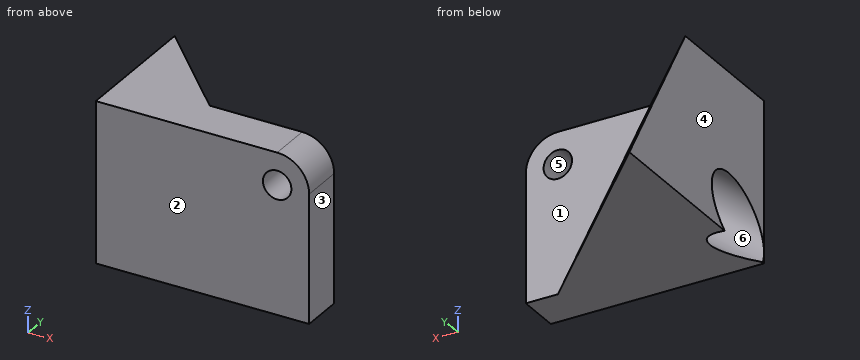
```python
from build123d import *

# Parameters (mm, degrees)
SKETCH_1_R          = 4
EXTRUDE_1_DEPTH     = 12
EXTRUDE_2_DEPTH     = 55
CUT_EXTRUDE_1_DEPTH = 50
SKETCH_9_R          = 9
CUT_EXTRUDE_2_DEPTH = 74.567594408


with BuildPart() as part:
    # 草图1 → 凸台-拉伸1 (new body)
    with BuildSketch(Plane(origin=(0, 0, 0), x_dir=(1, 0, 0), z_dir=(0, 1, 0))):
        with BuildLine():
            Line((-30, 22.5), (30, 22.5))
            Line((30, 22.5), (30, -13.5))
            ThreePointArc((30, -13.5), (27.363961031, -19.863961031), (21, -22.5))
            Line((21, -22.5), (-30, -22.5))
            Line((-30, -22.5), (-30, 22.5))
        make_face()
        with Locations(Location((21, -13.5, 0), (0, 0, 270))):
            Circle(SKETCH_1_R, mode=Mode.SUBTRACT)
    extrude(amount=EXTRUDE_1_DEPTH)

    # 草图5 → 凸台-拉伸2 (add)
    with BuildSketch(Plane(origin=(0, 12, 0), x_dir=(1, 0, 0), z_dir=(0, 1, 0))):
        Polygon((-5, -22.5), (20.980762114, 22.5), (-30, 22.5), (-30, -22.5), align=None)
    extrude(amount=EXTRUDE_2_DEPTH)

    # 草图6 → 切除-拉伸1 (cut)
    with BuildSketch(Plane(origin=(8.633922254, 8.365483215, 4.984797338), x_dir=(0.4999999999999977, 0, -0.86602540378444), z_dir=(-0.6634139481689368, -0.642787609686543, -0.3830222215594858))):
        Polygon((-21.985571585, -4.744524705), (29.975952642, -4.744524705), (46.861281787, -7.759213518), (18.600754365, -97.120116912), (-55.184549729, -73.785397471), align=None)
    extrude(amount=-CUT_EXTRUDE_1_DEPTH, mode=Mode.SUBTRACT)

    # 草图9 → 切除-拉伸2 (cut, through all)
    with BuildSketch(Plane(origin=(8.633922254, 8.365483215, 4.984797338), x_dir=(0.27508013503084955, 0.2665275624016649, -0.9237391286459811), z_dir=(0.663413948168937, 0.6427876096865428, 0.38302222155948573))):
        with Locations(Location((9.830913468, 29.914425108, 0), (0, 0, 90))):
            Circle(SKETCH_9_R)
    extrude(amount=-CUT_EXTRUDE_2_DEPTH, mode=Mode.SUBTRACT)


solid = part.part
```
Input: part model. Units: mm. Frame: model coordinates. Face numbers are marked on the shaded views. A direction names the side the tool comes from. Round coordinates to 2 decimals unless told otherwise and drop trailing zeros. Loops run counter-clockwise (first coordinate to the right, second up) from the corner with the lowest first, then second, coordinate; pieces in that order, holes last. Notation, with made-up numbers: M 50,81.5 L 101,81.5 A20 cw 101,108.5 Z; hole C -25,-1 d8. An arc over 180 degrees is marked long. Answer in a Markdown table with one row per item. Add a question column.
1. Ray query, probe 1 along X at (y, z) = (2.5, 13.5); probe 2 along Y at (x, z) = (25.5, 11); probe 3 along Z at (x, y) = (23.5, 3). Return the intervals inside material, ascending.
2. Section A-A (z = 5.5). Output: boundary loops of the cut face in (x, y), and give its area (3 significant figures).
3. Section B-B (y = 42). Output: boundary loops of the cut face in (x, z).
4. Contact query for flat-ended pins moving along their axis: pin 1 (5 mm diameter, centred on y = 7, z = -17.5, fed in from -X); pin 2 (4 mm diameter, centred on y = 27, z = -5.5, fed in from +X); pin 3 (8 mm diameter, centred on x = 8.5, z = -4, fed in from +Y). Output: stop coordinate, or through.
5. Mould query, pull axis X, two halves, no side actions, for the marked faces 3, 4, 5 and 6. Classes: released by +X, released by -X, zero draft, split by the parting line, or undercut.
6. Set-up query: the marked faces 1 and 2. Return all of +Z, -Z, +X, -X, +Y, -Y with unobstructed straight access to the full face (end or side cutting, diameter ignored); none if empty.
Values follow:
| question | item | result |
|---|---|---|
| 1 | probe 1 | -30 to 17, 25 to 30 |
| 1 | probe 2 | 0 to 12 |
| 1 | probe 3 | -22.5 to 10.38, 16.62 to 22.15 |
| 2 | outline | M -30,0 L 30,0 L 30,12 L 4.81,12 L -30,47.93 Z |
| 2 | area | 1,350 mm^2 |
| 3 | outline | M -30,-22.5 L -8.09,-22.5 L -30,15.46 Z |
| 4 | pin 1 | x = -25.45 |
| 4 | pin 2 | x = -1.11 |
| 4 | pin 3 | y = 18.62 |
| 5 | face 3 | released by +X |
| 5 | face 4 | released by -X |
| 5 | face 5 | undercut |
| 5 | face 6 | undercut |
| 6 | face 1 | +Z, +X, +Y |
| 6 | face 2 | +Z, -Z, +X, -X, -Y |
